Geometry: final body of the model. Coordinates: model frame, mm. Face numbers are marked on the shaded views. A direction names the side the tool comes from. Give positions to 0.01 mm unless a question says otherwise; leave off trailing zeros. Write each loop counter-clockwise with the first axis right and the second up, starting at its lowest first coordinate (ties: lowest second). Pieces come first, ordered by that corner, then holes.
Q1. Cut plane A-A on y = 16.74. Return the cut outline in (x, z).
Q2. Reachability of the marked faces 4, 5, 6 and 7 from +Z, -Z, +X, -X, +Y, -Y: full face, straight path, thin tool, end or side. Return the list, or none.
Q3. Pin query (flat end, axial travel): pin 1 (16 mm diameter, centred on y = 16.74, z = -21, fed in from +X); pin 2 (1.5 mm diameter, centred on x = 7, z = -3.5, fed in from +Y); pin 3 (9 mm diameter, centred on y = 23, z = -27.5, fed in from -X). Return the tip coordinate at first contact, or that it passes through.
Q4. Cut plane C-C on z = -17. Return the cut outline in (x, y), plus the area to 3 significant figures.
Q5. Cut plane D-D on x = 7.25. Return the cut outline in (y, z).
Q6. Cut plane B-B on x = 1.5. Return the cut outline in (y, z).
Q7. Line query: L1, parallel to Z at x = 5, y = 1.3; L2, parallel to Z at x = 7.65, y = 16.74; L3, parallel to Y at x = 7.6, z = -21. Output: solid intervals per line, ascending.
Q8. Draft query along Z for the marked faces 1, 2 and 3. Return one class per face: pulls with the +Z half, pulls with the -Z half, needs draft (parallel to the pull), parting line crosses it, or undercut.
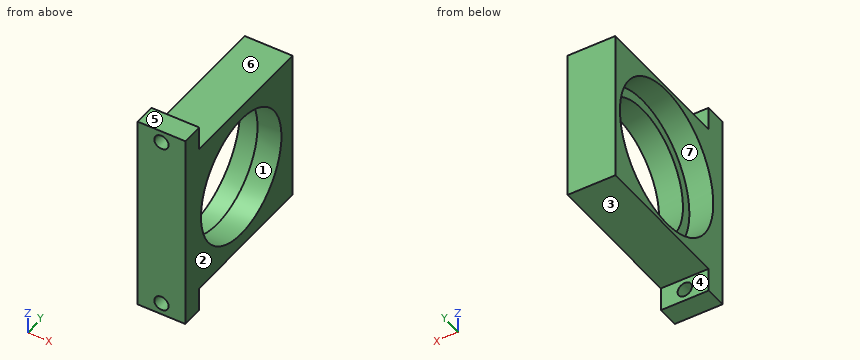
Autodesk Inventor part; units mm, degrees
ref_plane "Work Plane1" through (0, 0, -21) normal (0, 0, 1) x (1, 0, 0)
ref_plane "YZ Plane" through (0, 0, 0) normal (1, 0, 0) x (0, 1, 0)
ref_plane "XZ Plane" through (0, 0, 0) normal (0, 1, 0) x (-1, 0, 0)
sketch "Sketch1" plane through (0, 0, 0) normal (1, 0, 0) x (0, 1, 0)
  line L0 (0, 0) -> (33.48, 0)
  line L1 (33.48, 0) -> (33.48, -42)
  line L2 (33.48, -42) -> (0, -42)
  line L3 (0, -42) -> (0, 0)
  point P0 (33.48, -21)
  point P1 (16.74, 0)
  dimension "d0" = 33.48
  dimension "d1" = 42
extrude "Extrusion1" add sketch "Sketch1" along normal blind 10
sketch "Sketch2" plane through (10, 0, 0) normal (1, 0, 0) x (0, 0, -1)
  line L0 (0, 33.48) -> (0, 0)
  line L1 (42, 33.48) -> (0, 33.48)
  point P0 (21, 16.74)
  point P1 (0, 16.74)
  point P2 (21, 33.48)
hole "Hole1" at (10, 16.74, -21) direction (-1, 0, 0) diameter 26.289 depth 66.675 tip angle 118
sketch "Sketch3" plane through (0, 0, 0) normal (0, 0, 1) x (1, 0, 0)
  line L0 (0, 0) -> (0, 33.48)
  line L1 (0, 33.48) -> (10, 33.48)
  line L2 (0, 3) -> (10, 3)
  line L3 (10, 3) -> (10, 33.48)
  line L4 (10, 33.48) -> (0, 33.48)
  line L5 (0, 33.48) -> (0, 3)
  line L6 (0, 0) -> (10, 0)
  dimension "d12" = 3
extrude "Extrusion2" cut sketch "Sketch3" against normal blind 5
sketch "Sketch6" plane through (0, 0, -42) normal (0, -1, 0) x (1, 0, 0)
  line L0 (0, 42) -> (0, 0)
  line L1 (0, 0) -> (10, 0)
  line L2 (0, 42) -> (10, 42)
  line L3 (10, 42) -> (10, 0)
  line L4 (10, 0) -> (0, 0)
  line L5 (0, 0) -> (0, 42)
extrude "Extrusion3" add sketch "Sketch6" along normal blind 1.5
ref_plane "Work Plane1" through (0, 0, -21) normal (0, 0, 1) x (1, 0, 0)
sketch "Sketch4" plane through (0, 3, 0) normal (0, 1, 0) x (1, 0, 0)
  line L0 (10, 5) -> (10, 0)
  line L1 (10, 0) -> (0, 0)
  point P0 (5, 2.5)
  point P1 (10, 2.5)
  point P2 (5, 0)
hole "Hole2" at (5, 3, -2.5) direction (0, -1, 0) diameter 3 end through all
mirror "Mirror1" about plane through (0, 0, -21) normal (0, 0, 1) of "Hole2", "Extrusion2"
sketch "Sketch5" plane through (0, 0, 0) normal (-1, 0, 0) x (0, 0, 1)
  circle A0 centre (-21, 16.74) radius 13.1445
  point P0 (0, 0)
hole "Hole3" at (0, 16.74, -21) direction (1, 0, 0) diameter 30.48 depth 5
properties part number "Laser holder3" material "Aluminum 6061"
Data:
1. outline: (0, -37) - (10, -37) - (10, -34.14) - (5, -34.14) - (5, -36.24) - (0, -36.24) - close; (0, -5.76) - (5, -5.76) - (5, -7.86) - (10, -7.86) - (10, -5) - (0, -5) - close
2. face 4: -Z, +X, -X, +Y
2. face 5: +Z, +X, -X, +Y, -Y
2. face 6: +Z, +X, -X, +Y
2. face 7: -X
3. pin 1: passes through
3. pin 2: stops at y = 3
3. pin 3: stops at x = 5
4. outline: (0, -1.5) - (10, -1.5) - (10, 4.22) - (5, 4.22) - (5, 2.03) - (0, 2.03) - close; (0, 31.45) - (5, 31.45) - (5, 29.26) - (10, 29.26) - (10, 33.48) - (0, 33.48) - close
4. area: 77.5 mm2
5. outline: (-1.5, -42) - (3, -42) - (3, -37) - (33.48, -37) - (33.48, -5) - (3, -5) - (3, 0) - (-1.5, 0) - close; hole circle Ø26.29 at (16.74, -21)
6. outline: (-1.5, -42) - (3, -42) - (3, -37) - (33.48, -37) - (33.48, -5) - (3, -5) - (3, 0) - (-1.5, 0) - close; hole circle Ø30.48 at (16.74, -21)
7. L1: z = -42 to -41, -38 to -4, -1 to 0
7. L2: z = -37 to -34.14, -7.86 to -5
7. L3: y = -1.5 to 3.6, 29.88 to 33.48
8. face 1: undercut
8. face 2: needs draft
8. face 3: pulls with the -Z half
